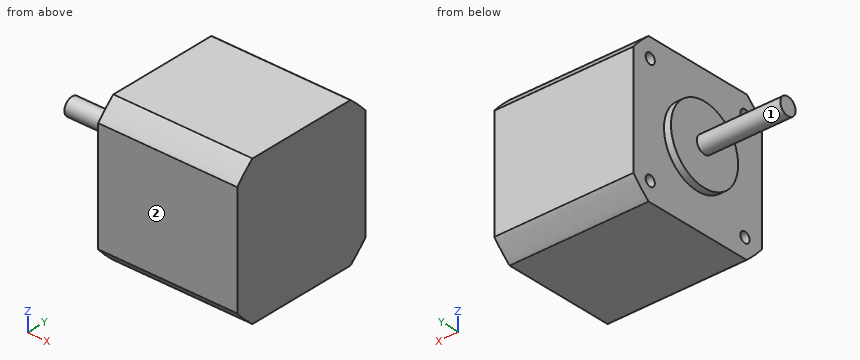
```python
from build123d import *

# Parameters (mm, degrees)
SKETCH1_W           = 42
SKETCH1_H           = 42
BOSS_EXTRUDE1_DEPTH = 40
SKETCH2_R           = 11
BOSS_EXTRUDE2_DEPTH = 2
SKETCH3_R           = 2.5
BOSS_EXTRUDE3_DEPTH = 24
SKETCH4_R           = 1.5
CUT_EXTRUDE1_DEPTH  = 4.5
FILLET1_SIZE        = 5


with BuildPart() as part:
    # Sketch1 → Boss-Extrude1 (new body)
    with BuildSketch(Plane(origin=(0, 0, 0), x_dir=(0, 0, -1), z_dir=(1, 0, 0))):
        with Locations((21, -21)):
            Rectangle(SKETCH1_W, SKETCH1_H)
    extrude(amount=BOSS_EXTRUDE1_DEPTH)

    # Sketch2 → Boss-Extrude2 (add)
    with BuildSketch(Plane.ZY):
        with Locations(Location((-21, -21, 0), (0, 0, 180))):
            Circle(SKETCH2_R)
    extrude(amount=BOSS_EXTRUDE2_DEPTH)

    # Sketch3 → Boss-Extrude3 (add)
    with BuildSketch(Plane.ZY.offset(2)):
        with Locations((-21, -21)):
            Circle(SKETCH3_R)
    extrude(amount=BOSS_EXTRUDE3_DEPTH)

    # Sketch4 → Cut-Extrude1 (cut)
    with BuildSketch(Plane.ZY):
        with Locations((-36.5, -5.5)):
            Circle(SKETCH4_R)
        with Locations((-5.5, -5.5)):
            Circle(SKETCH4_R)
        with Locations((-5.5, -36.5)):
            Circle(SKETCH4_R)
        with Locations((-36.5, -36.5)):
            Circle(SKETCH4_R)
    extrude(amount=-CUT_EXTRUDE1_DEPTH, mode=Mode.SUBTRACT)

    # Fillet1
    # a fillet whose section is not a circle: 5 mm, written as the material it takes off along each edge
    with BuildSketch(Plane(origin=(-12.5, -42, 0), x_dir=(0, 1, 0), z_dir=(1, 0, 0)), Plane(origin=(-12.5, 0, 0), x_dir=(0, 0, -1), z_dir=(1, 0, 0))) as fillet1_piece_1:
        with BuildLine():
            Bezier((FILLET1_SIZE, 0), (0, 0), (0, -FILLET1_SIZE), weights=[1, 0.052631579, 1])
            Line((0, -FILLET1_SIZE), (0, 0))
            Line((0, 0), (FILLET1_SIZE, 0))
        make_face()
    extrude(amount=65, mode=Mode.SUBTRACT)
    with BuildSketch(Plane(origin=(-12.5, -42, -42), x_dir=(0, 1, 0), z_dir=(1, 0, 0)), Plane(origin=(-12.5, 0, -42), x_dir=(0, 0, 1), z_dir=(1, 0, 0))) as fillet1_piece_2:
        with BuildLine():
            Bezier((FILLET1_SIZE, 0), (0, 0), (0, FILLET1_SIZE), weights=[1, 0.052631579, 1])
            Line((0, FILLET1_SIZE), (0, 0))
            Line((0, 0), (FILLET1_SIZE, 0))
        make_face()
    extrude(amount=65, mode=Mode.SUBTRACT)


solid = part.part
```
Could you check a few things on this model? Use its own coordinates, in mm. Face numbers are marked on the shaded views. A direction names the side the tool comes from. Round coordinates to 2 decimals unless told otherwise and drop trailing zeros. Order: outer loops, then holes, each group sorted by start corner. A loop starts at its lowest first (then second) coordinate and runs counter-clockwise, first axis right, second up. Notation, with made-up numbers: (60, 86.5) -> (72, 86.5) arc R36 ccw to (72, 125.5) -> close; hole circle Ø1 at (21, 71.25). An arc over 180 degrees is marked (long way). One line per question, with ' | ' between items.
Q1. If we section it at D-D on z = -16: Write out the boundary of the cut face in (x, y), plus the area to 3 significant figures.
Computed values:
outline: (-2, -30.8) -> (0, -30.8) -> (0, -42) -> (40, -42) -> (40, 0) -> (0, 0) -> (0, -11.2) -> (-2, -11.2) -> close | area: 1,720 mm²
Q2. If I drill on line 1 (Y direction, x = 3.15, z = -36.5); line 2 (Z direction, x = 3, y = -5), over which ranges is the centre line in solid material (lowest first)? Write a range as from..to.
Computed values:
line 1: -42..-38, -35..-7, -4..0 | line 2: -42..-37.91, -35.09..-6.91, -4.09..0
Q3. Which directions (+Z, -Z, +X, -X, +Y, -Y) give clear straight access to the entire face, cutting with the end or side of a thin tool? Please do the marked faces 1 and 2.
Computed values:
face 1: -X | face 2: +Z, -Z, +X, -X, -Y
Q4. If we section it at A-A on y = -21: Write out the boundary of the cut face in (x, z).
Computed values:
outline: (-26, -23.5) -> (-2, -23.5) -> (-2, -32) -> (0, -32) -> (0, -42) -> (40, -42) -> (40, 0) -> (0, 0) -> (0, -10) -> (-2, -10) -> (-2, -18.5) -> (-26, -18.5) -> close
Q5. If we section it at C-C on x = -11.5: Write out the boundary of the cut face in (y, z).
Computed values:
outline: circle Ø5 at (-21, -21)
Q6. I'm going to push flat-ended pins straight in: pin 1 (6 mm diameter, centred on x = -5.5, z = -23.5, fed in from +Y); pin 2 (10 mm diameter, centred on x = -10, z = -6.5, fed in from +Y); pin 3 (2.5 mm diameter, centred on y = -5, z = -37, fed in from -X); pin 4 (1.5 mm diameter, centred on y = -5.5, z = -6, fed in from -X). Where does each tip first touch, or does it pass through?
Computed values:
pin 1: y = -18.5 | pin 2: through | pin 3: x = 0 | pin 4: x = 4.5
